Here's how the part is built. I have some questions about the finished solid (model axes, mm). Round coordinates to 2 decimals unless told otherwise and drop trailing zeros. Write each loop counter-clockwise with the first axis right and the second up, starting at its lowest first coordinate (ties: lowest second). Pieces come first, ordered by that corner, then holes. Notation, with made-up numbers: M -35.5,-6.5 L 15.5,-6.5 A13 cw 15.5,13.5 Z; hole C 29,-24.5 d5. An arc over 180 degrees is marked long. Use one line per item in the form item = value. Start each with the question number.
Q1. We'd pull the mould along Y, two halves only. Please class faces 1 (the face through (-214.108, 411.648, -14.79)), 2 (the face through (-5.923, 45.113, -200.969)), 3 (the face through (-346, -311, 0)), 4 (the face through (61.2, 466, -15.2)): +Y half, -Y half, draft (parallel to the pull), parting line (faces both ways), or undercut.
Q2. I want a section at A-A on z = -14. List the corners of the cut face in (x, y) for me, and give its area (3 significant figures).
Q3. I need wall thicknesses on line 1 along X through (y, z) = (340.5, -20); line 2 along Y through (x, z) = (-242, -31.5); line 3 along Y through (x, z) = (341, -18). Which ranges of each line are inside material? Lowest first, please. Write a range as from..to.
Q4. I'm going to push flat-ended pins straight in: pin 1 Ø1 at (x, y) = (-137.5, 44.5) entering from -Z; pin 2 Ø3 at (y, z) = (-250, -60.5) entering from +X; pin 3 Ø1 at (x, y) = (104.5, 131.5) entering from -Z. Where does each tip first touch, or does it pass through?
Q5. I want a section at B-B on z = -104. List the corners of the cut face in (x, y) for me.
Autodesk Inventor part; units mm, degrees
ref_plane "YZ Plane" through (0, 0, 0) normal (1, 0, 0) x (0, 1, 0)
ref_plane "XZ Plane" through (0, 0, 0) normal (0, 1, 0) x (-1, 0, 0)
ref_plane "XY Plane" through (0, 0, 0) normal (0, 0, 1) x (1, 0, 0)
sketch "Sketch1" plane through (0, 0, 0) normal (0, 1, 0) x (-1, 0, 0)
  line L0 (470, 0) -> (470, -30)
  arc A0 (408.9405, -122.1066) -> (470, -30) centre (370, -30) ccw
  arc A1 (0, -205) -> (408.9405, -122.1066) centre (0, 845.1667) ccw
  line L1 (0, 191.6842) -> (0, -191.6842)
  arc A2 (0, -199) -> (406.6041, -116.5802) centre (0, 845.1667) ccw
  arc A3 (406.6041, -116.5802) -> (464, -30) centre (370, -30) ccw
  line L2 (464, -30) -> (464, 0)
  line L3 (464, 0) -> (470, 0)
  line L4 (0, -199) -> (0, -205)
  point P0 (0, 0)
  point P1 (0, 0)
  point P2 (0, -202)
  point P3 (0, -163.7009)
  point P4 (0, -169.7009)
  dimension "d0" = 100
  dimension "d1" = 30
  dimension "d3" = 1050.1667
  dimension "d6" = 6
  dimension "d11" = 928
  dimension "d12" = 205
revolve "Revolution1" add sketch "Sketch1" angle 360 about axis through (0, 0, 191.6842) along (0, 0, -1)
sketch "Sketch2" plane through (0, 0, 0) normal (0, 0, 1) x (1, 0, 0)
  circle A0 centre (0, 0) radius 45.5
  dimension "d8" = 91
extrude "Extrusion1" cut sketch "Sketch2" against normal through all
equation "\"d11\" = MAIN_filter_diam"
equation "\"MAIN_filter_diam\" = 928"
equation "\"Disherd_head_hight\" = d12"
properties part number "PRS 940-02 dished head" material "Steel"
Reported:
q1.face_1 = undercut
q1.face_2 = undercut
q1.face_3 = draft
q1.face_4 = parting line
q2.outline = C 0,0 d940; hole C 0,0 d928
q2.area = 17,600 mm^2
q3.line_1 = -323.97..-315.21, 315.21..323.97
q3.line_2 = -402.9..-395.88, 395.88..402.9
q3.line_3 = -323.45..-314.67, 314.67..323.45
q4.pin_1 = -195.08
q4.pin_2 = 393.46
q4.pin_3 = -191.56
q5.outline = C 0,0 d874.52; hole C 0,0 d855.93
